Model file for the job. Use its own axes, mm. A direction names the side the tool comes from. Round coordinates to 2 decimals unless told otherwise and drop trailing zeros. Order: outer loops, then holes, each group sorted by start corner. A loop starts at its lowest first (then second) coordinate and runs counter-clockwise, first axis right, second up. Notation, with made-up numbers: (-18.75, 9) - (-2.75, 9) arc R25 ccw to (-2.75, 33) - close; hole circle Ø6 at (85.25, 31). An arc over 180 degrees is marked (long way). Write item = value, one per line.
```python
from build123d import *

# Parameters (mm, degrees)
F0_W      = 25.4
F0_H      = 3.175
F1_DEPTH  = 25.4
F2_W      = 3.175
F2_H      = 15.24
F3_DEPTH  = 25.4
F5_D      = 3.2639
F5_DEPTH  = 12.7
F5_TIP    = 0.9805744872
F7_D      = 3.2639
F7_DEPTH  = 12.7
F7_TIP    = 0.9805744872
F8_W      = 25.4
F8_H      = 3.175
F9_DEPTH  = 3.176
F11_DEPTH = 3.176


with BuildPart() as f1:
    # F0 (on Front) → F1 (new body)
    with BuildSketch(Plane.XZ):
        with Locations((13.8182396877, 1.5875)):
            Rectangle(F0_W, F0_H)
    extrude(amount=F1_DEPTH)

    # F2 (on face) → F3 (join)
    with BuildSketch(Plane.YZ.offset(26.5182396877)):
        with Locations((-23.8125, 10.795)):
            Rectangle(F2_W, F2_H)
    extrude(amount=-F3_DEPTH)

    # F5
    with Locations(Plane(origin=(0, -22.225, 0), x_dir=(-1, 0, 0), z_dir=(0, 1, 0))):
        with Locations((-20.1682396877, 10.795), (-7.4682396877, 10.795)):
            Hole(F5_D / 2, depth=F5_DEPTH)
            with Locations((0, 0, -(F5_DEPTH + F5_TIP / 2))):  # 118° drill point
                Cone(0, F5_D / 2, F5_TIP, mode=Mode.SUBTRACT)

    # F7
    with Locations(Plane.XY.offset(3.175)):
        with Locations((7.4682396877, -14.605), (20.1682396877, -14.605)):
            Hole(F7_D / 2, depth=F7_DEPTH)
            with Locations((0, 0, -(F7_DEPTH + F7_TIP / 2))):  # 118° drill point
                Cone(0, F7_D / 2, F7_TIP, mode=Mode.SUBTRACT)

    # F8 (on face) → F9 (cut, through all)
    with BuildSketch(Plane(origin=(0, -22.225, 0), x_dir=(-1, 0, 0), z_dir=(0, 1, 0))):
        with Locations((-13.8182396877, 16.8275)):
            Rectangle(F8_W, F8_H)
    extrude(amount=-F9_DEPTH, mode=Mode.SUBTRACT)

    # F10 (on face) → F11 (cut, through all)
    with BuildSketch(Plane.XY.offset(3.175)):
        Polygon((13.8182396877, 0), (1.1182396877, 0), (1.1182396877, -7.62), (26.5182396877, -7.62), (26.5182396877, 0), align=None)
    extrude(amount=-F11_DEPTH, mode=Mode.SUBTRACT)


solid = f1.part
```
1) Cut at C-C (y = -24). Write the cut outline in (x, z) (3 decimals).
Conclusion:
outline = (1.118, 0) - (26.518, 0) - (26.518, 15.24) - (1.118, 15.24) - close; hole circle Ø3.264 at (7.468, 10.795); hole circle Ø3.264 at (20.168, 10.795)
2) Cut at B-B (x = 20.75). Write the cut outline in (y, z) (3 decimals).
Conclusion:
outline = (-25.4, 0) - (-16.13, 0) - (-16.13, 3.175) - (-22.225, 3.175) - (-22.225, 9.27) - (-25.4, 9.27) - close; (-25.4, 12.32) - (-22.225, 12.32) - (-22.225, 15.24) - (-25.4, 15.24) - close; (-13.08, 0) - (-7.62, 0) - (-7.62, 3.175) - (-13.08, 3.175) - close
3) Mould opens along Z. For faces 1 (the face through (14, -15, 3.175)), 2 (the face through (6.173, -23.835, 9.802)), 3 (the face through (14, -25.4, 8)) say: +Z half, -Z half, draft (parallel to the pull), parting line (faces both ways), or undercut.
Conclusion:
face_1 = +Z half
face_2 = undercut
face_3 = draft
4) 3-axis set-ups, long thin cutter, end or side, ignore diameter. For faces 4 (the face through (14, -22.225, 9)), 5 (the face through (26.518, -21, 3)): which of +Z, -Z, +X, -X, +Y, -Y reach the whole face in a straight line?
Conclusion:
face_4 = +Z, +X, -X, +Y
face_5 = +Z, -Z, +X, +Y, -Y
5) Wall check: line 1 along Y through (x, z) = (24.5, 10.75) (3 decimals); line 2 along Z through (x, y) = (15.25, -9.5) (3 decimals); line 3 along Z through (x, y) = (20.75, -22.75). Give the ranges that are in metal, low to high.
Conclusion:
line_1 = -25.4 to -22.225
line_2 = 0 to 3.175
line_3 = 0 to 9.27, 12.32 to 15.24
6) Flat gauge pins, fed straight in: pin 1 Ø5 at (x, z) = (7.47, 10.8) entering from +Y (3 decimals); pin 2 Ø5 at (y, z) = (-18, 6.5) entering from +X; pin 3 Ø4 at (x, y) = (22.5, -12) entering from +Z (3 decimals). Where does each tip first touch, or does it go through?
Conclusion:
pin_1 = -22.225
pin_2 = through
pin_3 = 3.175
7) Cut at D-D (z = 1.75). Write the cut outline in (x, y) (3 decimals), and give its area (3 significant figures).
Conclusion:
outline = (1.118, -25.4) - (26.518, -25.4) - (26.518, -7.62) - (1.118, -7.62) - close; hole circle Ø3.264 at (7.468, -14.605); hole circle Ø3.264 at (20.168, -14.605)
area = 435 mm^2
8) Cut at A-A (z = 9.5). Write the cut outline in (x, y) (3 decimals).
Conclusion:
outline = (1.118, -25.4) - (6.475, -25.4) - (6.475, -22.225) - (1.118, -22.225) - close; (8.461, -25.4) - (19.175, -25.4) - (19.175, -22.225) - (8.461, -22.225) - close; (21.161, -25.4) - (26.518, -25.4) - (26.518, -22.225) - (21.161, -22.225) - close
